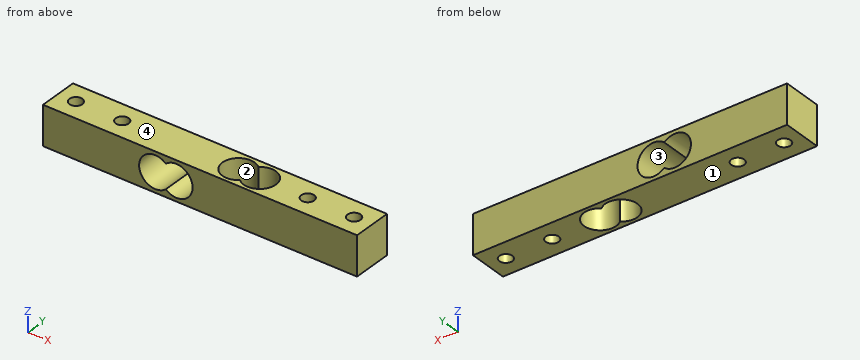
```python
from build123d import *

# Parameters (mm, degrees)
SKETCH1_W                 = 12.7
SKETCH1_H                 = 12.7
BOSS_EXTRUDE1_DEPTH       = 50.8
SKETCH2_R                 = 5.21
CUT_EXTRUDE1_DEPTH        = 101.6
SKETCH3_R                 = 5.21
CUT_EXTRUDE2_DEPTH        = 101.6
M5X0_8_TAPPED_HOLE2_D     = 4.2
M5X0_8_TAPPED_HOLE2_DEPTH = 14
M5X0_8_TAPPED_HOLE2_TIP   = 1.2618073


with BuildPart() as part:
    # Sketch1 → Boss-Extrude1 (new, symmetric)
    with BuildSketch(Plane(origin=(0, 0, 0), x_dir=(0, 0, -1), z_dir=(1, 0, 0))):
        Rectangle(SKETCH1_W, SKETCH1_H)
    extrude(amount=BOSS_EXTRUDE1_DEPTH, both=True)

    # Sketch2 → Cut-Extrude1 (cut)
    with BuildSketch(Plane(origin=(0, 6.35, 0), x_dir=(1, 0, 0), z_dir=(0, 1, 0))):
        with Locations((-7.62, 0)):
            Circle(SKETCH2_R)
        with Locations((-14.5, 0)):
            Circle(SKETCH2_R)
    extrude(amount=-CUT_EXTRUDE1_DEPTH, mode=Mode.SUBTRACT)

    # Sketch3 → Cut-Extrude2 (cut)
    with BuildSketch(Plane(origin=(0, 0, -6.35), x_dir=(-1, 0, 0), z_dir=(0, 0, -1))):
        with Locations((-14.5, 0)):
            Circle(SKETCH3_R)
        with Locations((-7.62, 0)):
            Circle(SKETCH3_R)
    extrude(amount=-CUT_EXTRUDE2_DEPTH, mode=Mode.SUBTRACT)

    # M5x0.8 Tapped Hole2
    with Locations(Plane(origin=(0, 0, -6.35), x_dir=(-1, 0, 0), z_dir=(0, 0, -1))):
        with Locations((-45, 0), (-30, 0), (30, 0), (45, 0)):
            Hole(M5X0_8_TAPPED_HOLE2_D / 2, depth=M5X0_8_TAPPED_HOLE2_DEPTH)
            with Locations((0, 0, -(M5X0_8_TAPPED_HOLE2_DEPTH + M5X0_8_TAPPED_HOLE2_TIP / 2))):  # 118° drill point
                Cone(0, M5X0_8_TAPPED_HOLE2_D / 2, M5X0_8_TAPPED_HOLE2_TIP, mode=Mode.SUBTRACT)


solid = part.part
```
The model under review builds one solid part; all positions refer to its coordinate system, in mm. Face numbers are marked on the shaded views. Coordinates: 2 decimals unless noted, no trailing zeros. Write each loop counter-clockwise with the first axis right and the second up, starting at its lowest first coordinate (ties: lowest second). Pieces come first, ordered by that corner, then holes.
1) We need section B-B on x = 7.62. State the section outline as (y, z) points.
2) The part is to be moulded in two halves that separate along Z. For the marked faces 1, 2, 3 and 4, say which applies: pulls with the +Z half, pulls with the -Z half, needs draft (parallel to the pull), parting line crosses it, or undercut.
3) To check wall thickness, follow probe 1 along Y at (x, z) = (30, 3.75); probe 2 along Y at (x, z) = (7.62, 3.5); probe 3 along X at (y, z) = (4.75, -1.5). State the ranges of each line that lie inside material, in increasing order.
4) We need section A-A on z = -1.5. State the section outline as (x, y) points, then the cut area to 3 significant figures.
5) We need section C-C on x = -45. State the section outline as (y, z) points, then the cut area to 3 significant figures.
Answer list:
1. outline: (-6.35, -6.35) - (-5.21, -6.35) - (-5.21, 6.35) - (-6.35, 6.35) - close; (5.21, -6.35) - (6.35, -6.35) - (6.35, 6.35) - (5.21, 6.35) - close
2. face 1: pulls with the -Z half
2. face 2: needs draft
2. face 3: undercut
2. face 4: pulls with the +Z half
3. probe 1: y = -6.35 to -2.1, 2.1 to 6.35
3. probe 2: y = -6.35 to -5.21, 5.21 to 6.35
3. probe 3: x = -50.8 to -19.49, -2.63 to 5.48, 9.76 to 12.36, 16.64 to 50.8
4. outline: (-50.8, -6.35) - (-19.49, -6.35) - (-19.49, 6.35) - (-50.8, 6.35) - close; (-2.63, -6.35) - (50.8, -6.35) - (50.8, 6.35) - (-2.63, 6.35) - close; hole circle Ø4.2 at (-45, 0); hole circle Ø4.2 at (-30, 0); hole (11.06, -3.91) arc R5.21 ccw (long way) to (11.06, 3.91) arc R5.21 ccw (long way) to start; hole circle Ø4.2 at (30, 0); hole circle Ø4.2 at (45, 0)
4. area: 869 mm2
5. outline: (-6.35, -6.35) - (-2.1, -6.35) - (-2.1, 6.35) - (-6.35, 6.35) - close; (2.1, -6.35) - (6.35, -6.35) - (6.35, 6.35) - (2.1, 6.35) - close
5. area: 108 mm2
